The listing builds one solid part. Answer for the finished solid, in the listing's coordinates (mm). A direction names the side the tool comes from. Give positions to 0.01 mm unless a question says otherwise; leave off trailing zeros. Order: outer loops, then holes, each group sorted by start corner. A loop starts at its lowest first (then second) coordinate and runs counter-clockwise, first axis right, second up.
```python
from build123d import *

# Parameters (mm, degrees)
SKETCH_1_W          = 327.6
SKETCH_1_H          = 253.6
EXTRUDE_1_DEPTH     = 15
SHELL_1_T           = -1.2
SKETCH_2_R          = 4.5
CUT_EXTRUDE_1_DEPTH = 15


with BuildPart() as part:
    # 草图1 → 凸台-拉伸1 (new body)
    with BuildSketch(Plane.XY):
        Rectangle(SKETCH_1_W, SKETCH_1_H)
    extrude(amount=EXTRUDE_1_DEPTH)

    # 抽壳1
    shell_1_openings = [part.faces().sort_by_distance(p)[0] for p in [
        (0, 0, 0),
    ]]
    offset(amount=SHELL_1_T, openings=shell_1_openings, kind=Kind.INTERSECTION)

    # 草图2 → 切除-拉伸1 (cut)
    with BuildSketch(Plane.XY.offset(15)):
        with Locations((-148.8, 111.8)):
            Circle(SKETCH_2_R)
        with Locations(Location((148.8, 111.8, 0), (0, 0, 180))):
            Circle(SKETCH_2_R)
        with Locations((148.8, -111.8)):
            Circle(SKETCH_2_R)
        with Locations(Location((-148.8, -111.8, 0), (0, 0, 180))):
            Circle(SKETCH_2_R)
    extrude(amount=-CUT_EXTRUDE_1_DEPTH, mode=Mode.SUBTRACT)


solid = part.part
```
1) A tool of negligible diameter and unlimited length cuts with its end or side. For faces 5 (the cylindrical face through (-144.64, 110.08, 14.41)), 6 (the flat face through (-162.6, -2, 7)), from which of +Z, -Z, +X, -X, +Y, -Y can it reach the whole face along a straight path? Write none if from no direction.
Geometry says:
face 5: +Z, -Z
face 6: -Z
2) Straight lines are drawn through the part: probe 1 along Y at (x, z) = (148.8, 14.35); probe 2 along Y at (x, z) = (37, 2); probe 3 along X at (y, z) = (43, 12.25). For each, find the intervals that lie inside material, in ascending order.
Geometry says:
probe 1: y = -126.8 to -116.3, -107.3 to 107.3, 116.3 to 126.8
probe 2: y = -126.8 to -125.6, 125.6 to 126.8
probe 3: x = -163.8 to -162.6, 162.6 to 163.8
3) Find section B-B (x = 148.8). Write down the section's boundary in (y, z).
Geometry says:
outline: (-126.8, 0) - (-125.6, 0) - (-125.6, 13.8) - (-116.3, 13.8) - (-116.3, 15) - (-126.8, 15) - close; (-107.3, 13.8) - (107.3, 13.8) - (107.3, 15) - (-107.3, 15) - close; (116.3, 13.8) - (125.6, 13.8) - (125.6, 0) - (126.8, 0) - (126.8, 15) - (116.3, 15) - close
4) Find section A-A (y = -111.8). Write down the section's boundary in (x, z).
Geometry says:
outline: (-163.8, 0) - (-162.6, 0) - (-162.6, 13.8) - (-153.3, 13.8) - (-153.3, 15) - (-163.8, 15) - close; (-144.3, 13.8) - (144.3, 13.8) - (144.3, 15) - (-144.3, 15) - close; (153.3, 13.8) - (162.6, 13.8) - (162.6, 0) - (163.8, 0) - (163.8, 15) - (153.3, 15) - close
5) Given P1, Ø1, axis at x = 98.5, y = -57, coming from the -Z side; P2, Ø5.5, axis at x = 148.8, y = -111.8, coming from the +Z side, each flat-ended and moving along its own axis, determine where each tip first touches the part or whether it passes through.
Geometry says:
P1: stops at z = 13.8
P2: passes through
6) For a pull along Y with two mould halves and no side action, classify faces 1 (the cylindrical face through (144.64, 113.52, 14.41)), 2 (the flat face through (-163.8, -2, 7)), 3 (the flat face through (-2, -126.8, 7)), 4 (the flat face through (-2, 2, 13.8)) as +Y half, -Y half, draft (parallel to the pull), parting line (faces both ways), or undercut.
Geometry says:
face 1: undercut
face 2: draft
face 3: -Y half
face 4: undercut
7) Find section D-D (y = -28.5). Write down the section's boundary in (x, z), then the cut area to 3 significant figures.
Geometry says:
outline: (-163.8, 0) - (-162.6, 0) - (-162.6, 13.8) - (162.6, 13.8) - (162.6, 0) - (163.8, 0) - (163.8, 15) - (-163.8, 15) - close
area: 426 mm2
8) Find section C-C (z = 9.5). Write down the section's boundary in (x, y).
Geometry says:
outline: (-163.8, -126.8) - (163.8, -126.8) - (163.8, 126.8) - (-163.8, 126.8) - close; hole (-162.6, -125.6) - (162.6, -125.6) - (162.6, 125.6) - (-162.6, 125.6) - close
